Part model, mm, in its own coordinate system. A direction names the side the tool comes from. Coordinates: 2 decimals unless noted, no trailing zeros. Loops run counter-clockwise (first coordinate to the right, second up) from the corner with the lowest first, then second, coordinate; pieces in that order, holes last. Notation, with made-up numbers: (28, 22.25) -> (51, 22.25) arc R26 ccw to (51, 50.25) -> close; hole circle Ø10 at (16, -33). An arc over 180 degrees is marked (long way). One line per item, written item: value. Start each with the question number.
Autodesk Inventor part; units mm, degrees
ref_plane "YZ Plane" through (0, 0, 0) normal (1, 0, 0) x (0, 1, 0)
ref_plane "XZ Plane" through (0, 0, 0) normal (0, 1, 0) x (-1, 0, 0)
ref_plane "XY Plane" through (0, 0, 0) normal (0, 0, 1) x (1, 0, 0)
sketch "Sketch1" plane through (0, 0, 0) normal (0, 0, 1) x (1, 0, 0)
  arc A0 (0, -25.4) -> (0, 25.4) centre (0, 0) ccw
  line L0 (0, 25.4) -> (0, 44.45)
  line L1 (0, 44.45) -> (38.1, 44.45)
  line L2 (38.1, 44.45) -> (38.1, -44.45)
  line L3 (38.1, -44.45) -> (0, -44.45)
  line L4 (0, -44.45) -> (0, -25.4)
  dimension "d1" = 44.45
  dimension "d2" = 38.1
  dimension "d3" = 88.9
  dimension "d4" = 25.4
extrude "Extrusion1" add sketch "Sketch1" along normal mid plane 12.7
sketch "Sketch2" plane through (0, 0, 6.35) normal (0, 0, 1) x (1, 0, 0)
  line L0 (38.1, -44.45) -> (38.1, 44.45)
  line L1 (38.1, 26.67) -> (27.2088, 26.67)
  line L2 (38.1, 44.45) -> (0, 44.45)
  line L3 (38.1, -26.67) -> (27.2088, -26.67)
  line L4 (0, -44.45) -> (38.1, -44.45)
  arc A0 (27.2088, -26.67) -> (27.2088, 26.67) centre (0, 0) ccw
  point P0 (38.1, 0)
  dimension "d7" = 17.78
  dimension "d9" = 38.1
extrude "Extrusion2" cut sketch "Sketch2" against normal through all
sketch "Sketch3" plane through (0, 0, 0) normal (0, 0, 1) x (1, 0, 0)
  arc A0 (0, -31.75) -> (0, 31.75) centre (0, 0) ccw
  arc A1 (0, -25.4) -> (0, 25.4) centre (0, 0) ccw
  line L0 (0, 25.4) -> (0, 31.75)
  line L1 (0, 25.4) -> (0, 44.45)
  line L2 (0, -25.4) -> (0, -31.75)
  line L3 (0, -44.45) -> (0, -25.4)
  line L4 (0, 25.4) -> (0, 31.75)
  line L5 (0, -31.75) -> (0, -25.4)
  dimension "d14" = 31.75
extrude "Extrusion3" add sketch "Sketch3" along normal mid plane 19.05
fillet "Fillet1" radius 3.175 2 edges at (27.2088, -26.67, 0) (27.2088, 26.67, 0)
fillet "Fillet2" radius 6.35 4 edges at (19.05, 44.45, 6.35) (19.05, 44.45, -6.35) (19.05, -44.45, 6.35) (19.05, -44.45, -6.35)
sketch "Sketch4" plane through (38.1, -26.67, 6.35) normal (1, 0, 0) x (0, 0, -1)
  circle A0 centre (6.35, 64.77) radius 3.175
  circle A1 centre (6.35, -11.43) radius 3.175
  arc A2 (0, -11.43) -> (12.7, -11.43) centre (6.35, -11.43) ccw
  arc A3 (12.7, 64.77) -> (0, 64.77) centre (6.35, 64.77) ccw
  point P0 (6.35, 26.67)
  dimension "d19" = 6.35
extrude "Extrusion4" cut sketch "Sketch4" against normal through all
properties part number "rodcap"
1) Pin check, flat tips, straight feed: pin 1 Ø4 at (x, z) = (33, -4.5) entering from +Y; pin 2 Ø1 at (x, z) = (17.5, -4) entering from -Y. Stop position of each tip, or through.
2) Slice it at A-A (x = 21.5). State how many separate pieces and enclosed holes the cut face has, then the cut area to 3 significant figures.
3) Pull direction Z, two halves, no side cores. Call faces 1 (the cylindrical face through (18.78, -42.54, -4.54)), 2 (the flat face through (31, 9, 6.35)), 3 (the cylindrical face through (19.32, 35, 0.69)), 4 (the flat face through (0, -33, 0)): +Z half, -Z half, draft (parallel to the pull), parting line (faces both ways), or undercut.
4) Slice it at D-D (z = 7.5). Give the cut face in (x, y), then the cut area to 3 significant figures.
5) Tool access for faces 5 (the flat face through (36, -26.67, 0)), 6 (the flat face through (31, 9, -6.35)), 7 (the cylindrical face through (31.742, 0.698, 7.915)): list every direction of +Z, -Z, +X, -X, +Y, -Y with a clear straight run to the whole face (end or side of a thin tool).
6) Slice it at C-C (y = 20.5). Give the cut face in (x, z) (3 decimals), then the cut area to 3 significant figures.
7) Slice it at B-B (z = 1). Give the cut face in (x, y) (3 decimals), then the cut area to 3 significant figures.
8) Probe line 1 (Y direction, x = 17, z = 0) (3 decimals); line 2 (Y direction, x = 22, z = 1.5); line 3 (Y direction, x = 29.5, z = 2.75). List the from-to ranges inside material, lowest first. Write a range as from..to.
Check sheet entries:
1. pin 1: stops at y = 43.94
1. pin 2: stops at y = -43.4
2. separate pieces: 2
2. enclosed holes: 2
2. area: 813 mm^2
3. face 1: -Z half
3. face 2: +Z half
3. face 3: undercut
3. face 4: draft
4. outline: (0, -31.75) arc R31.75 ccw to (0, 31.75) -> (0, 25.4) arc R25.4 cw to (0, -25.4) -> close
4. area: 570 mm^2
5. face 5: +Z, -Z, +X
5. face 6: -Z, +X
5. face 7: +Z, +X
6. outline: (14.997, -9.525) -> (24.245, -9.525) -> (24.245, -6.35) -> (32.115, -6.35) -> (32.115, 6.35) -> (24.245, 6.35) -> (24.245, 9.525) -> (14.997, 9.525) -> close
6. area: 276 mm^2
7. outline: (0, -44.371) -> (38.1, -44.371) -> (38.1, -41.113) -> (0, -41.113) -> close; (0, -35.087) -> (38.1, -35.087) -> (38.1, -26.67) -> (33.935, -26.67) arc R3.175 cw to (31.325, -21.688) arc R38.1 ccw to (31.325, 21.688) arc R3.175 cw to (33.935, 26.67) -> (38.1, 26.67) -> (38.1, 35.087) -> (0, 35.087) -> (0, 25.4) arc R25.4 cw to (0, -25.4) -> close; (0, 41.113) -> (38.1, 41.113) -> (38.1, 44.371) -> (0, 44.371) -> close
7. area: 1,750 mm^2
8. line 1: y = -44.45..-41.275, -34.925..-18.872, 18.872..34.925, 41.275..44.45
8. line 2: y = -44.27..-40.9, -35.3..-12.69, 12.69..35.3, 40.9..44.27
8. line 3: y = -43.82..-39.69, -36.51..36.51, 39.69..43.82
